```python
from build123d import *

# Parameters (mm, degrees)
SKETCH1_W           = 11
SKETCH1_H           = 8.5
BOSS_EXTRUDE1_DEPTH = 75
SKETCH14_W          = 11
SKETCH14_H          = 8.5
FILLET1_R           = 10
BOSS_EXTRUDE3_START = -8.5
BOSS_EXTRUDE3_DEPTH = 8.5
FILLET5_R           = 10
FILLET6_R           = 5
SKETCH18_R          = 1.25
BOSS_EXTRUDE4_DEPTH = 1.5
SKETCH19_R          = 1.25
BOSS_EXTRUDE5_DEPTH = 1.5
REVOLVE9_ANGLE      = 180
REVOLVE10_ANGLE     = 180


with BuildPart() as part:
    # Sketch1 → Boss-Extrude1 (new body)
    with BuildSketch(Plane(origin=(0, 0, 0), x_dir=(0, 0, -1), z_dir=(1, 0, 0))):
        with Locations((5.5, -4.25)):
            Rectangle(SKETCH1_W, SKETCH1_H)
    extrude(amount=BOSS_EXTRUDE1_DEPTH)

    # Sweep3: sweep along a curve in space
    with BuildLine() as sweep3_path:
        Line((75, -3, -5.5), (85, -3, -5.5))
        Line((85, -3, -5.5), (99.142135624, 11.142135624, -5.5))
        Line((99.142135624, 11.142135624, -5.5), (119.142135624, 11.142135624, -5.5))
    # Sketch14 → Sweep3 (sweep)
    with BuildSketch(Plane(origin=(75, 0, 0), x_dir=(0, 0, -1), z_dir=(1, 0, 0))):
        with Locations((5.5, -4.25)):
            Rectangle(SKETCH14_W, SKETCH14_H)
    sweep(path=sweep3_path.line, transition=Transition.RIGHT)

    # Fillet1
    fillet1_edges = [part.edges().sort_by_distance(p)[0] for p in [
        (97.899494937, 14.142135624, -5.5),
        (101.420310217, 5.642135624, -5.5),
        (83.757359313, 0, -5.5),
        (87.278174593, -8.5, -5.5),
    ]]
    fillet(fillet1_edges, radius=FILLET1_R)

    # Sketch17 → Boss-Extrude3 (add)
    with BuildSketch(Plane(origin=(0, 0, 0), x_dir=(1, 0, 0), z_dir=(0, 1, 0)).offset(BOSS_EXTRUDE3_START)):
        with BuildLine():
            Line((-10, -10), (-13.5, -10))
            Line((-13.5, -10), (-13.5, -13.5))
            Line((-13.5, -13.5), (-10, -13.5))
            ThreePointArc((-10, -13.5), (-0.454058454, -9.545941546), (3.5, 0))
            Line((3.5, 0), (3.5, 11))
            ThreePointArc((3.5, 11), (-0.454058454, 20.545941546), (-10, 24.5))
            Line((-10, 24.5), (-13.5, 24.5))
            Line((-13.5, 24.5), (-13.5, 21))
            Line((-13.5, 21), (-10, 21))
            ThreePointArc((-10, 21), (-2.928932188, 18.071067812), (0, 11))
            Line((0, 11), (0, 0))
            ThreePointArc((0, 0), (-2.928932188, -7.071067812), (-10, -10))
        make_face()
    extrude(amount=BOSS_EXTRUDE3_DEPTH)

    # Fillet5
    fillet5_edges = [part.edges().sort_by_distance(p)[0] for p in [
        (3.5, -4.25, 0),
        (3.5, -4.25, -11),
    ]]
    fillet(fillet5_edges, radius=FILLET5_R)

    # Fillet6
    # the kernel refuses this fillet: 5 mm, written as the material it takes off along each edge
    with BuildSketch(Plane(origin=(-13.5, -8.5, -2.5), x_dir=(0, 1, 0), z_dir=(0, 0, 1)), Plane(origin=(-13.5, 0, -2.5), x_dir=(1, 0, 0), z_dir=(0, 0, 1)), Plane(origin=(-13.5, -8.5, -37), x_dir=(0, 1, 0), z_dir=(0, 0, 1)), Plane(origin=(-13.5, 0, -37), x_dir=(1, 0, 0), z_dir=(0, 0, 1))) as fillet6_piece_1:
        with BuildLine():
            CenterArc((FILLET6_R, -FILLET6_R), FILLET6_R, 90, 90)
            Line((0, -FILLET6_R), (0, 0))
            Line((0, 0), (FILLET6_R, 0))
        make_face()
    extrude(amount=28.5, mode=Mode.SUBTRACT)

    # Sketch18 → Boss-Extrude4 (add)
    with BuildSketch(Plane.XY.offset(-21)):
        with Locations(Location((-10, -5, 0), (0, 0, 270))):
            Circle(SKETCH18_R)
    extrude(amount=BOSS_EXTRUDE4_DEPTH)

    # Sketch19 → Boss-Extrude5 (add)
    with BuildSketch(Plane(origin=(0, 0, 10), x_dir=(-1, 0, 0), z_dir=(0, 0, -1))):
        with Locations(Location((10, -3.5, 0), (0, 0, 269.999999996))):
            Circle(SKETCH19_R)
    extrude(amount=BOSS_EXTRUDE5_DEPTH)

    # Sketch24 → Revolve9 (revolve)
    with BuildSketch(Plane(origin=(0, 0, 8.5), x_dir=(-1, 0, 0), z_dir=(0, 0, -1))):
        with BuildLine():
            Line((10, -2.25), (10, -4.75))
            ThreePointArc((10, -4.75), (11.25, -3.5), (10, -2.25))
        make_face()
    revolve(axis=Axis((-10, -2.25, 8.5), (0, -1, 0)), revolution_arc=REVOLVE9_ANGLE)

    # Sketch25 → Revolve10 (revolve)
    with BuildSketch(Plane.XY.offset(-19.5)):
        with BuildLine():
            Line((-10, -3.75), (-10, -6.25))
            ThreePointArc((-10, -6.25), (-11.25, -5), (-10, -3.75))
        make_face()
    revolve(axis=Axis((-10, -3.75, -19.5), (0, 1, 0)), revolution_arc=REVOLVE10_ANGLE)


solid = part.part
```
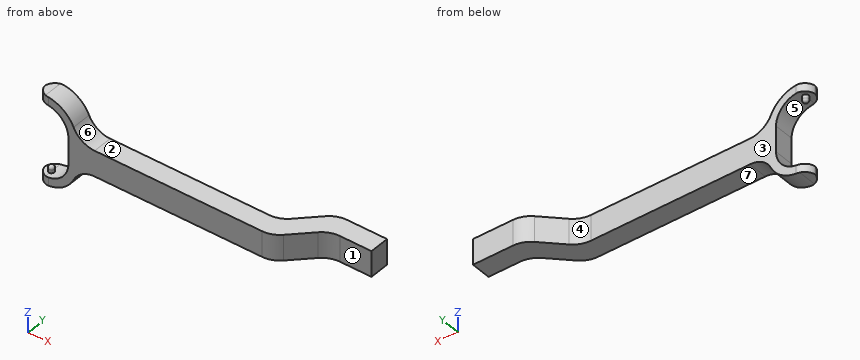
Input: part model. Units: mm. Frame: model coordinates. Face numbers are marked on the shaded views. A direction names the side the tool comes from. Give positions to 0.01 mm unless a question says otherwise; leave off trailing zeros. Order: outer loops, then holes, each group sorted by start corner. A loop starts at its lowest first (then second) coordinate and runs counter-clockwise, first axis right, second up.
1. Cut plane C-C (y = 7.5). Return loops of the section in (x, z), and give its area (3 significant figures).
Computed:
outline: (91.26, -11) - (119.14, -11) - (119.14, 0) - (91.26, 0) - close
area: 307 mm2
2. Draft query along Z for the marked faces 4, 5, 6 and 7. Return one class per face: released by +Z, released by -Z, zero draft, split by the parting line, or undercut.
Computed:
face 4: zero draft
face 5: undercut
face 6: released by +Z
face 7: released by -Z
3. Set-up query: the marked faces 1, 2 and 3. Return all of +Z, -Z, +X, -X, +Y, -Y with unobstructed straight access to the full face (end or side cutting, diameter ignored); none if empty.
Computed:
face 1: +Z, -Z, +X, -Y
face 2: +Z, +X, +Y, -Y
face 3: +Z, -Z, -X, +Y
4. Pin query (flat end, axial travel): pin 1 Ø4 at (y, z) = (-3, -3) entering from -X; pin 2 Ø10 at (x, z) = (88.5, -8.5) entering from +Y; pin 3 Ø7 at (x, y) = (87, 0) entering from +Z. Return the tip coordinate at first contact, or that it passes through.
Computed:
pin 1: stops at x = 0
pin 2: stops at y = 9.74
pin 3: stops at z = 0
5. Cut plane B-B (x = 75.5). Return loops of the section in (y, z), and give its area (3 significant figures).
Computed:
outline: (-8.5, -11) - (0, -11) - (0, 0) - (-8.5, 0) - close
area: 93.5 mm2
6. Line query: probe 1 along Z at (x, y) = (89, -5); probe 2 along X at (y, z) = (8.75, -8.5); probe 3 along Y at (x, z) = (16.5, -1). Output: solid intervals per line, ascending.
Computed:
probe 1: z = -11 to 0
probe 2: x = 92.51 to 119.14
probe 3: y = -8.5 to 0
7. Cut plane A-A (z = -3.5). Return loops of the section in (x, y).
Computed:
outline: (0, -8.5) - (83.14, -8.5) arc R10 ccw to (90.21, -5.57) - (98.49, 2.71) arc R10 cw to (105.56, 5.64) - (119.14, 5.64) - (119.14, 14.14) - (102.04, 14.14) arc R10 ccw to (94.97, 11.21) - (86.69, 2.93) arc R10 cw to (79.62, 0) - (0, 0) - close
